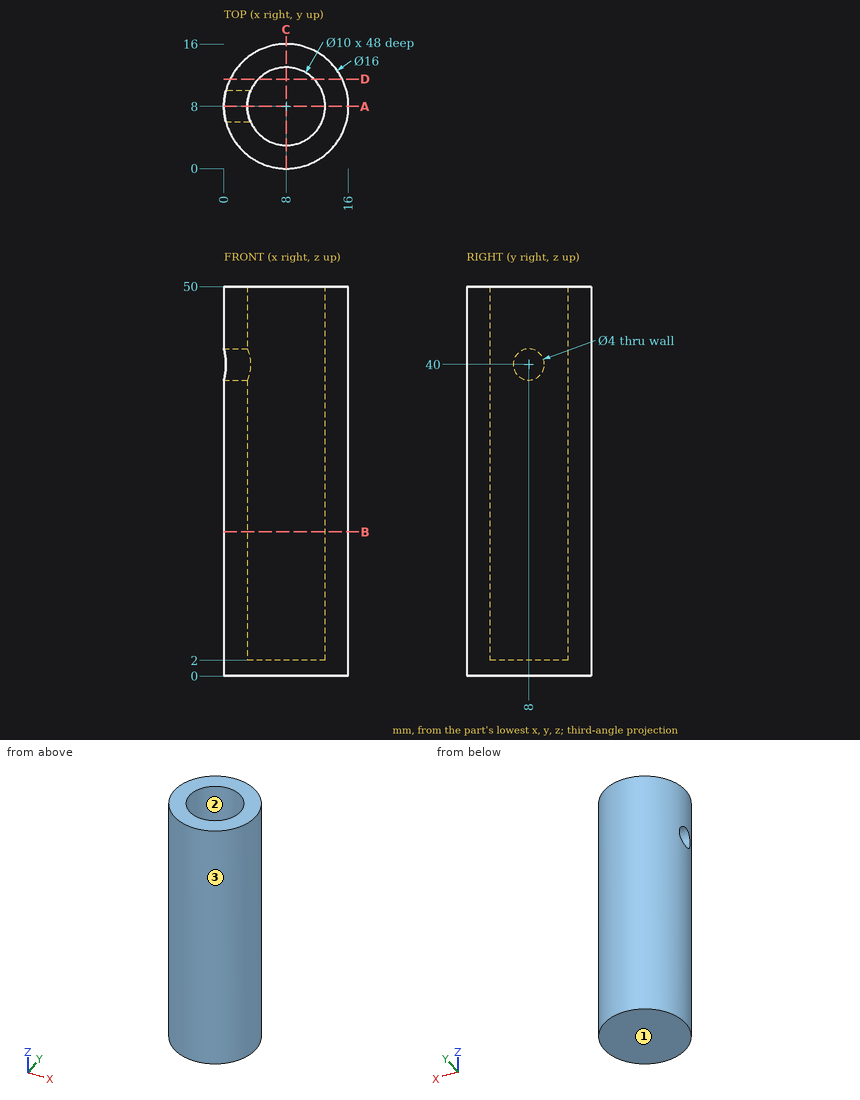
Drawing for the job (mm, zero at the part's lowest x, y, z). Round coordinates to 2 decimals unless told otherwise and drop trailing zeros. Loops run counter-clockwise (first coordinate to the right, second up) from the corner with the lowest first, then second, coordinate; pieces in that order, holes last. Notation, with made-up numbers: (78, 51.25) -> (109, 51.25) arc R26 ccw to (109, 80.25) -> close; hole circle Ø4 at (-34, 38). An arc over 180 degrees is marked (long way). Answer as CSV lines item,"result". Start each with the question number.
1) Slice it at C-C (x = 8). List the corners of the cut face in (y, z), plus the area to 3 significant figures.
2) Pin check, flat tips, straight feed: P1, Ø1.5, axis at y = 5.5, z = 36.5, coming from the -X side; P2, Ø1, axis at x = 9, z = 39, coming from the +Y side; P3, Ø5, axis at x = 2.5, z = 7, coming from the +Y side. Stop position of each tip, or through.
3) Slice it at B-B (z = 18.5). List the corners of the cut face in (x, y).
4) Probe line 1 along Y through (x, z) = (8, 12.5); line 2 along Z through (x, y) = (5.25, 8); line 3 along X through (y, z) = (8.5, 5). List the from-to ranges inside material, lowest first.
5) Mould opens along X. For the marked faces 1, 2 and 3 say: +X half, -X half, draft (parallel to the pull), parting line (faces both ways), or undercut.
6) Slice it at D-D (y = 11.5). List the corners of the cut face in (x, z), plus the area to 3 significant figures.
7) Slice it at A-A (y = 8). List the corners of the cut face in (x, z), plus the area to 3 significant figures.
Filled in:
1,outline,"(0, 0) -> (16, 0) -> (16, 50) -> (13, 50) -> (13, 2) -> (3, 2) -> (3, 50) -> (0, 50) -> close"
1,area,"320 mm2"
2,P1,"stops at x = 0.19"
2,P2,"stops at y = 15.98"
2,P3,"stops at y = 15.42"
3,outline,"circle Ø16 at (8, 8); hole circle Ø10 at (8, 8)"
4,line 1,"y = 0 to 3, 13 to 16"
4,line 2,"z = 0 to 2"
4,line 3,"x = 0.02 to 3.03, 12.97 to 15.98"
5,face 1,"draft"
5,face 2,"undercut"
5,face 3,"parting line"
6,outline,"(0.81, 0) -> (15.19, 0) -> (15.19, 50) -> (11.57, 50) -> (11.57, 2) -> (4.43, 2) -> (4.43, 50) -> (0.81, 50) -> close"
6,area,"377 mm2"
7,outline,"(0, 0) -> (16, 0) -> (16, 50) -> (13, 50) -> (13, 2) -> (3, 2) -> (3, 38) -> (0, 38) -> close; (0, 42) -> (3, 42) -> (3, 50) -> (0, 50) -> close"
7,area,"308 mm2"
